Input: part model. Units: mm. Frame: model coordinates. Face numbers are marked on the shaded views. Coordinates: 2 decimals unless noted, no trailing zeros. Order: outer loops, then holes, each group sorted by start corner. A loop starts at its lowest first (then second) coordinate and runs counter-clockwise, first axis right, second up. Notation, with made-up numbers: (34.5, 14.25) - (63.5, 14.25) arc R27 ccw to (63.5, 31.25) - close; hole circle Ø10 at (46, 64.5). An arc over 180 degrees is marked (long way). Use a Markdown table: item, result. Add a question column.
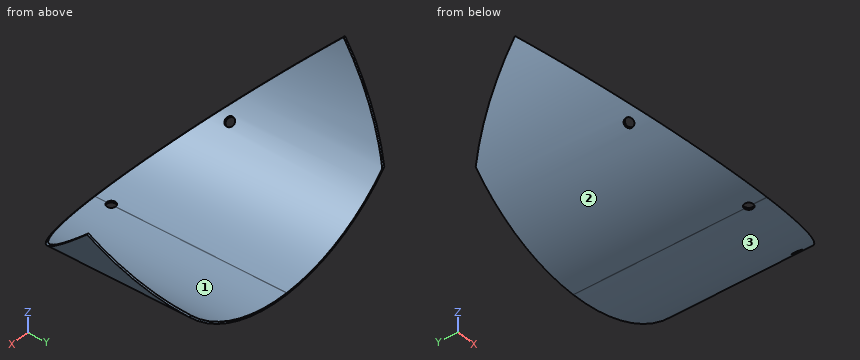
from build123d import *

# Parameters (mm, degrees)
SKETCH1_W                       = 0.254
SKETCH1_H                       = 152.4
BASE_FLANGE1_DEPTH              = 1.29032
EDGE_FLANGE1_DEPTH              = 152.4
EDGE_FLANGE1_BEND_DEPTH         = 152.4
CUT_EXTRUDE6_DEPTH              = 229.952357039
CUT_EXTRUDE6_DEPTH_BACK         = 229.952357039
SKETCH15_R                      = 3.175
CUT_EXTRUDE7_DEPTH              = 208.900927137
CIRPATTERN2_COUNT               = 2
CIRPATTERN2_ANGLE               = 52
CIRPATTERN2_THE_OTHER_WAY_COUNT = 2
CIRPATTERN2_THE_OTHER_WAY_ANGLE = 52


# Sheet-metal steps are written as plain solids
with BuildPart() as part:
    # Sketch1 → Base-Flange1 (new body)
    with BuildSketch(Plane.XY):
        with Locations((0, 76.2)):
            Rectangle(SKETCH1_W, SKETCH1_H)
    extrude(amount=-BASE_FLANGE1_DEPTH)

    # Edge-Flange1 section (across the edge) → Edge-Flange1 (add)
    with BuildSketch(Plane(origin=(114.427, 0, 0), x_dir=(-1, 0, 0), z_dir=(0, 1, 0))):
        with BuildLine():
            Line((-1.29032, 114.3), (-1.29032, 125.70968))
            Line((-1.29032, 125.70968), (0, 125.70968))
            Line((0, 125.70968), (0, 114.3))
            ThreePointArc((0, 114.3), (33.47769491, 33.47769491), (114.3, 0))
            Line((114.3, 0), (114.3, -1.29032))
            ThreePointArc((114.3, -1.29032), (32.565300888, 32.565300888), (-1.29032, 114.3))
        make_face()
    extrude(amount=EDGE_FLANGE1_DEPTH)

    # Edge-Flange1 section 2 (across the edge) → Edge-Flange1 bend (add)
    with BuildSketch(Plane(origin=(-114.427, 152.4, 0), x_dir=(1, 0, 0), z_dir=(0, -1, 0))):
        with BuildLine():
            Line((-1.29032, 114.3), (-1.29032, 125.70968))
            Line((-1.29032, 125.70968), (0, 125.70968))
            Line((0, 125.70968), (0, 114.3))
            ThreePointArc((0, 114.3), (33.47769491, 33.47769491), (114.3, 0))
            Line((114.3, 0), (114.3, -1.29032))
            ThreePointArc((114.3, -1.29032), (32.565300888, 32.565300888), (-1.29032, 114.3))
        make_face()
    extrude(amount=EDGE_FLANGE1_BEND_DEPTH)

    # Sketch14 → Cut-Extrude6 (cut, two sides: drawn at the far end of the back side and taken through both)
    with BuildSketch(Plane(origin=(0, 0, 0), x_dir=(0, 0, -1), z_dir=(1, 0, 0)).offset(-CUT_EXTRUDE6_DEPTH_BACK)):
        Polygon((-85.086344518, 102.789769459), (40.691860392, -22.988435452), (-72.437884386, -136.118180231), (-256.114134731, 47.558070115), (-142.984389953, 160.687814893), (-68.759425458, 243.273840802), (-6.680849316, 181.19526466), align=None)
    extrude(amount=CUT_EXTRUDE6_DEPTH + CUT_EXTRUDE6_DEPTH_BACK, mode=Mode.SUBTRACT)

    # Sketch15 → Cut-Extrude7 (cut, symmetric)
    with BuildSketch(Plane(origin=(0, 0, -1.29032), x_dir=(-1, 0, 0), z_dir=(0, 0, -1))):
        with Locations(Location((0.127, 29.11310494, 0), (0, 0, 90))):
            Circle(SKETCH15_R)
    cut_extrude7 = extrude(amount=CUT_EXTRUDE7_DEPTH, both=True, mode=Mode.SUBTRACT)

    # CirPattern2: Cut-Extrude7 ×2 about axis
    cirpattern2_axis = Axis((0, 79.569647195, 79.569647195), (0, 0.707106781186544, -0.7071067811865511))
    for i in range(1, CIRPATTERN2_COUNT):
        add(cut_extrude7.rotate(cirpattern2_axis, i * CIRPATTERN2_ANGLE / (CIRPATTERN2_COUNT - 1)), mode=Mode.SUBTRACT)

    # CirPattern2 the other way: Cut-Extrude7 ×2 about axis
    cirpattern2_the_other_way_axis = Axis((0, 79.569647195, 79.569647195), (0, -0.707106781186544, 0.7071067811865511))
    for i in range(1, CIRPATTERN2_THE_OTHER_WAY_COUNT):
        add(cut_extrude7.rotate(cirpattern2_the_other_way_axis, i * CIRPATTERN2_THE_OTHER_WAY_ANGLE / (CIRPATTERN2_THE_OTHER_WAY_COUNT - 1)), mode=Mode.SUBTRACT)


solid = part.part
1) Cut plane D-D (x = 47). Return the cut outline in (y, z), and give its area (3 significant figures).
2) Material intervals for L1, parallel to X at y = 83.5, z = 16.5; L2, parallel to X at y = 57.5, z = 26.5; L3, parallel to Z at x = -16, y = 125.5, sorted ascending.
3) Cut plane B-B (z = 40). Return the cut outline in (x, y).
4) Contact query for flat-ended pins moving along their axis: P1, Ø4, axis at x = -69.5, y = 74.5, coming from the +Z side; P2, Ø8, axis at x = 60, y = 82.5, coming from the -Z side; P3, Ø10, axis at x = 66, y = 102.5, coming from the -Z side. Output: stop coordinate, or through.
5) Cut plane A-A (y = 30). Return the cut outline in (x, z).
6) Pull-direction query (X, two-part tool) for the marked faces 1, 2 and 3; classes: pulls with the +X half, pulls with the -X half, needs draft (parallel to the pull), parting line crosses it, or undercut.
7) Cut plane C-C (y = 130). Return the cut outline in (x, z).
Computed:
| question | item | result |
|---|---|---|
| 1 | outline | (26.34, 8.64) - (152.4, 8.64) - (152.4, 10.05) - (27.76, 10.05) - close |
| 1 | area | 177 mm2 |
| 2 | L1 | x = -61.74 to -59.28, 59.28 to 61.74 |
| 2 | L2 | x = -75.31 to -73.31, 73.31 to 75.31 |
| 2 | L3 | z = -0.2 to 1.11 |
| 3 | outline | (-88.67, 57.7) - (-86.98, 57.7) - (-86.98, 147.88) - (-88.67, 147.88) - close; (86.98, 57.7) - (88.67, 57.7) - (88.67, 147.88) - (86.98, 147.88) - close |
| 4 | P1 | stops at z = 25.02 |
| 4 | P2 | stops at z = 13.11 |
| 4 | P3 | stops at z = 16.04 |
| 5 | outline | (-54.5, 12.3) arc R115.59 ccw to (-3.18, -1.25) - (-3.18, 0.04) arc R114.3 cw to (-51.7, 12.3) - close; (2.92, -1.26) arc R115.59 ccw to (54.5, 12.3) - (51.7, 12.3) arc R114.3 cw to (2.92, 0.03) - close |
| 6 | face 1 | undercut |
| 6 | face 2 | pulls with the -X half |
| 6 | face 3 | pulls with the +X half |
| 7 | outline | (-101.01, 57.88) arc R115.59 ccw to (-0.13, -1.29) - (0.13, -1.29) arc R115.59 ccw to (101.01, 57.88) - (99.53, 57.88) arc R114.3 cw to (0.13, 0) - (-0.13, 0) arc R114.3 cw to (-99.53, 57.88) - close |
